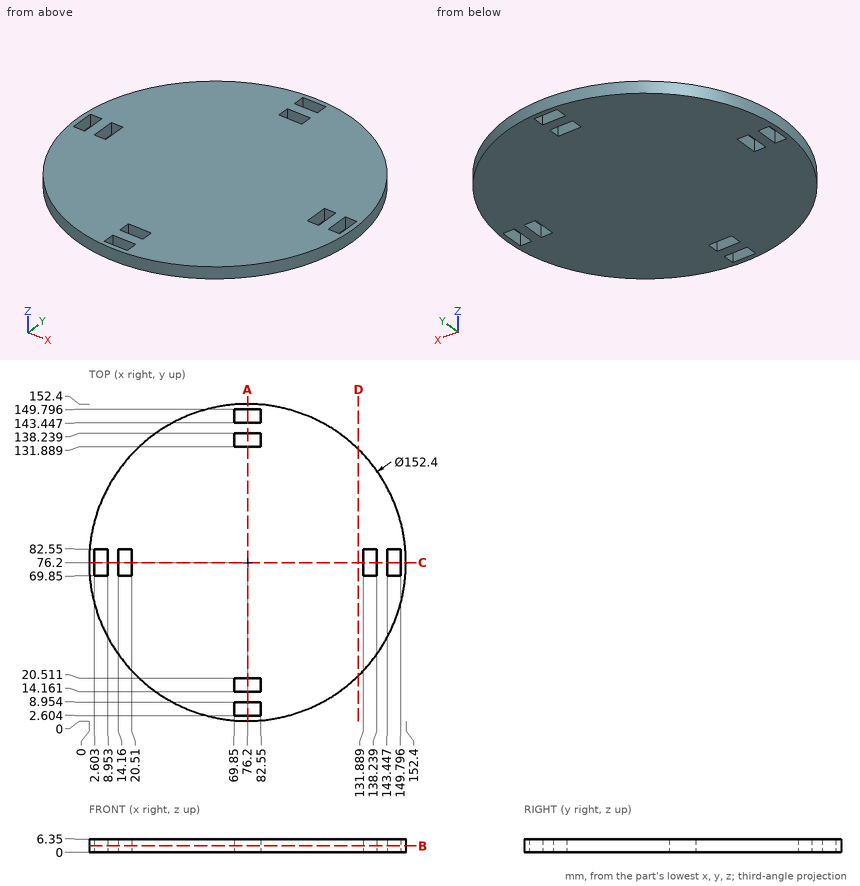
Part print with two shaded views. Sizes in mm from the minimum x, y, z corner. Give positions to 0.01 mm unless a question says otherwise; leave off trailing zeros. Write each loop counter-clockwise with the first axis right and the second up, starting at its lowest first coordinate (ties: lowest second). Pieces come first, ordered by that corner, then holes.
1) Cut at A-A on x = 76.2. Write the cut outline in (y, z).
Resolved:
outline: (0, 0) - (2.6, 0) - (2.6, 6.35) - (0, 6.35) - close; (8.95, 0) - (14.16, 0) - (14.16, 6.35) - (8.95, 6.35) - close; (20.51, 0) - (131.89, 0) - (131.89, 6.35) - (20.51, 6.35) - close; (138.24, 0) - (143.45, 0) - (143.45, 6.35) - (138.24, 6.35) - close; (149.8, 0) - (152.4, 0) - (152.4, 6.35) - (149.8, 6.35) - close
2) Pin check, flat tips, straight feed: pin 1 (3 mm diameter, centred on y = 19, z = 1.5, fed in from -X); pin 2 (3 mm diameter, centred on x = 92, z = 4, fed in from +Y); pin 3 (1 mm diameter, centred on x = 65.5, z = 4, fed in from +Y). Stop position of each tip, or through.
Resolved:
pin 1: stops at x = 24.2
pin 2: stops at y = 151.05
pin 3: stops at y = 151.71
3) Cut at D-D on x = 129.5. Write the cut outline in (y, z).
Resolved:
outline: (21.74, 0) - (130.66, 0) - (130.66, 6.35) - (21.74, 6.35) - close
4) Probe L1, parallel to X at y = 74, z = 4.25; L2, parallel to Y at x = 71.5, z = 0.5 (1 decimal); L3, parallel to Y at x = 68, z = 4.5. List the from-to ranges inside material, lowest first.
Resolved:
L1: x = 0.03 to 2.6, 8.95 to 14.16, 20.51 to 131.89, 138.24 to 143.45, 149.8 to 152.37
L2: y = 0.1 to 2.6, 9 to 14.2, 20.5 to 131.9, 138.2 to 143.4, 149.8 to 152.3
L3: y = 0.44 to 151.96
5) Cut at B-B on z = 3. State how many separate pieces and enclosed holes the cut face has, then the cut area to 3 significant figures.
Resolved:
separate pieces: 1
enclosed holes: 8
area: 17,600 mm2
